Design review of the part built by this model. Coordinates are the model's own, in mm. Face numbers are marked on the shaded views. A direction names the side the tool comes from. Round coordinates to 2 decimals unless told otherwise and drop trailing zeros. Write each loop counter-clockwise with the first axis right and the second up, starting at its lowest first coordinate (ties: lowest second). Pieces come first, ordered by that corner, then holes. Notation, with made-up numbers: M -14,77 L 36,77 A20 cw 36,100 Z; hole C -25.75,66.25 d4. An arc over 180 degrees is marked long. Use CSV: the item, a comma, the result in double quotes.
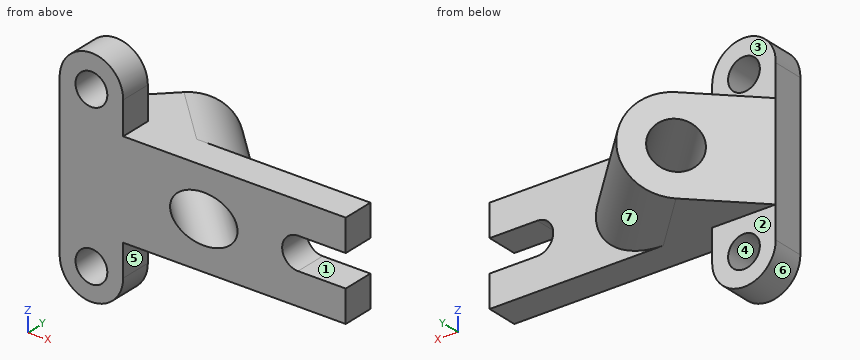
from build123d import *

# Parameters (mm, degrees)
BOSS_EXTRUDE2_DEPTH = 20
SKETCH2_R           = 10
CUT_EXTRUDE1_DEPTH  = 174.204794268
BOSS_EXTRUDE3_REACH = 201.499
CUT_EXTRUDE3_REACH  = 204.653
SKETCH5_R           = 15
CUT_EXTRUDE4_DEPTH  = 182.107428775


with BuildPart() as part:
    # Sketch1 → Boss-Extrude2 (new body)
    with BuildSketch(Plane(origin=(0, 0, 0), x_dir=(1, 0, 0), z_dir=(0, 1, 0))):
        with BuildLine():
            Line((0, 60), (140, 60))
            Line((140, 60), (140, 0))
            Line((140, 0), (0, 0))
            Line((0, 0), (0, -20.563630546))
            ThreePointArc((0, -20.563630546), (-20.285292958, -40.565119434), (-39.999007572, -20.000048944))
            Line((-39.999007572, -20.000048944), (-39.999007572, 80))
            ThreePointArc((-39.999007572, 80), (-19.999503786, 99.999503786), (0, 80))
            Line((0, 80), (0, 60))
        make_face()
    extrude(amount=BOSS_EXTRUDE2_DEPTH)

    # Sketch2 → Cut-Extrude1 (cut, through all)
    with BuildSketch(Plane(origin=(0, 20, 0), x_dir=(1, 0, 0), z_dir=(0, 1, 0))):
        with Locations(Location((-19.999503786, 80, 0), (0, 0, 270))):
            Circle(SKETCH2_R)
        with Locations(Location((-19.999503786, -20.000048944, 0), (0, 0, 270))):
            Circle(SKETCH2_R)
    extrude(amount=-CUT_EXTRUDE1_DEPTH, mode=Mode.SUBTRACT)

    # Boss-Extrude3: up to this face of the body (flat: up to its plane)
    boss_extrude3_end = Plane(part.part.faces().sort_by_distance((37.926780592, 20, -29.884787344))[0])
    # Sketch4 → Boss-Extrude3 (add, up to the picked face)
    with BuildSketch(Plane(origin=(-29.999503786, 29.999503786, 0), x_dir=(0, 0, 1), z_dir=(-0.7071067811865488, 0.7071067811865464, 0)), mode=Mode.PRIVATE) as boss_extrude3_sk1:
        with BuildLine():
            Line((-60, -14.141433871), (-60, 35.858566129))
            ThreePointArc((-60, 35.858566129), (-30, 65.858566129), (0, 35.858566129))
            Line((0, 35.858566129), (0, -14.141433871))
            Line((0, -14.141433871), (-60, -14.141433871))
        make_face()
    boss_extrude3_tool1 = split(extrude(boss_extrude3_sk1.sketch, amount=-BOSS_EXTRUDE3_REACH, mode=Mode.PRIVATE), bisect_by=boss_extrude3_end, keep=Keep.BOTH, mode=Mode.PRIVATE)
    add(boss_extrude3_tool1.solids().sort_by(Axis((-13.775448, 46.22356, -30), (0.7071067811865488, -0.7071067811865464, 0)))[0])

    # Cut-Extrude3: up to this plane
    cut_extrude3_end = Plane(origin=(-20.003474187, 0, 20.563630546), z_dir=(0, 1, 0))
    # Sketch5 → Cut-Extrude3 (cut, up to the surface)
    with BuildSketch(Plane(origin=(-29.999503786, 29.999503786, 0), x_dir=(0, 0, 1), z_dir=(-0.7071067811865487, 0.7071067811865465, 0)), mode=Mode.PRIVATE) as cut_extrude3_sk1:
        with Locations(Location((-30, 35.858566129, 0), (0, 0, 270))):
            Circle(SKETCH5_R)
    cut_extrude3_tool1 = split(extrude(cut_extrude3_sk1.sketch, amount=-CUT_EXTRUDE3_REACH, mode=Mode.PRIVATE), bisect_by=cut_extrude3_end, keep=Keep.BOTH, mode=Mode.PRIVATE)
    add(cut_extrude3_tool1.solids().sort_by_distance((-4.643669, 55.355339, -30))[0], mode=Mode.SUBTRACT)

    # Sketch6 → Cut-Extrude4 (cut, through all)
    with BuildSketch(Plane(origin=(0, 20, 0), x_dir=(1, 0, 0), z_dir=(0, 1, 0))):
        with BuildLine():
            Line((140, 40), (110, 40))
            ThreePointArc((110, 40), (100, 30), (110, 20))
            Line((110, 20), (140, 20))
            Line((140, 20), (140, 40))
        make_face()
    extrude(amount=-CUT_EXTRUDE4_DEPTH, mode=Mode.SUBTRACT)


solid = part.part
1) Add section B-B on z = -64.5. Write out the cut boundary in (x, y), then the cut area to 3 significant figures.
Answers:
outline,"M -40,0 L 0,0 L 0,20 L -40,20 Z"
area,"800 mm²"
2) The part is to be moulded in two halves that separate along Z. For the marked faces 4, 5, 6 and 7, say which applies: released by +Z, released by -Z, zero draft, split by the parting line, or undercut.
Answers:
face 4,"undercut"
face 5,"zero draft"
face 6,"released by -Z"
face 7,"split by the parting line"
3) Add section C-C on x = 79. Write out the cut boundary in (y, z).
Answers:
outline,"M 0,-60 L 20,-60 L 20,0 L 0,0 Z"
4) Add section D-D on z = -10. Write out the cut boundary in (x, y).
Answers:
outline,"M -40,0 L 140,0 L 140,20 L 62.33,20 L 11.17,71.17 L -40,20 Z"
5) For pin 1 Ø22 at (y, z) = (5.5, -36) entering from -X; pin 2 Ø8 at (y, z) = (38.5, -5) entering from -X; pin 3 Ø1.5 at (y, z) = (48, -42) entering from +X; pin 4 Ø12 at (x, z) = (-20, -80) entering from +Y, all flat-tipped, find the tip position at first contact; note any pin that passes through.
Answers:
pin 1,"x = -40"
pin 2,"x = -25.5"
pin 3,"x = 42.47"
pin 4,"through"
6) Add section A-A on z = -25.5. Write out the cut boundary in (x, y), then the cut area to 3 significant figures.
Answers:
outline,"M -40,0 L 30.48,0 L -14.76,45.24 L -40,20 Z; M 5.47,65.47 L 70.95,0 L 101.07,0 L 101.07,20 L 72.66,20 L 16.33,76.33 Z"
area,"3,750 mm²"
7) Wall thickness on line 1 along Z through (x, y) = (125.5, 11); line 2 along X through (y, z) = (10, -80); line 3 along Y through (x, z) = (97.5, -31.5): over which ranges is each line inside the solid? List them lowest first. Write a range as [from, to].
Answers:
line 1,"[-60, -40], [-20, 0]"
line 2,"[-40, -30], [-10, 0]"
line 3,"[0, 20]"
8) Machinability: for the marked faces 1, 2 and 3, which of the approach directions +Z, -Z, +X, -X, +Y, -Y give a long, thin tool a straight path to every point of the face, cutting with its end or side? Answer none if there is none.
Answers:
face 1,"+X, +Y, -Y"
face 2,"-Z, +X, -X, +Y"
face 3,"+Z, +X, -X, +Y"
